Input: part model. Units: mm. Frame: model coordinates. A direction names the side the tool comes from. Round coordinates to 2 decimals unless told otherwise and drop trailing zeros. Put each result on its own line as item: value. Start each with the question number.
1) Reachability of faces 1 (the face through (80, 38.2, -14)), 2 (the face through (137.5, 1, -14)) from +Z, -Z, +X, -X, +Y, -Y: full face, straight path, thin tool, end or side. Return the list, or none.
2) Draft query along Y for faces 3 (the face through (2, 1, -19.5)), 4 (the face through (-80, 41.8, -14)), 5 (the face through (-134.49, 57.15, -13.58)), 6 (the face through (134.49, -57.15, -13.58)). Return one class per face: +Y half, -Y half, draft (parallel to the pull), parting line (faces both ways), or undercut.
3) Line query: probe 1 along Y at (x, z) = (20, -9.75); probe 2 along Y at (x, z) = (80, -16.5); probe 3 along X at (y, z) = (-41, -11.75). Output: solid intervals per line, ascending.
from build123d import *

# Parameters (mm, degrees)
SKETCH001_R  = 1.8
PAD001_DEPTH = 12


with BuildPart() as part:
    # Sketch001 → Pad001 (new body)
    with BuildSketch(Plane.XY.offset(-19.5)):
        with BuildLine():
            Line((-127.5, 60), (127.5, 60))
            ThreePointArc((137.5, 49.999999), (134.571068, 57.071067), (127.5, 60))
            Line((137.5, 49.999999), (137.5, -49.999999))
            ThreePointArc((127.5, -60), (134.571068, -57.071067), (137.5, -49.999999))
            Line((127.5, -60), (-127.5, -60))
            ThreePointArc((-137.5, -50), (-134.571068, -57.071067), (-127.5, -60))
            Line((-137.5, -50), (-137.5, 50))
            ThreePointArc((-127.5, 60), (-134.571068, 57.071068), (-137.5, 50))
        make_face()
        with Locations((-80, -40)):
            Circle(SKETCH001_R, mode=Mode.SUBTRACT)
        with Locations((-50, -40)):
            Circle(SKETCH001_R, mode=Mode.SUBTRACT)
        with Locations((50, -40)):
            Circle(SKETCH001_R, mode=Mode.SUBTRACT)
        with Locations((80, -40)):
            Circle(SKETCH001_R, mode=Mode.SUBTRACT)
        with Locations((-127.5, -50)):
            Circle(SKETCH001_R, mode=Mode.SUBTRACT)
        with Locations((-127.5, 50)):
            Circle(SKETCH001_R, mode=Mode.SUBTRACT)
        with Locations((127.5, 50)):
            Circle(SKETCH001_R, mode=Mode.SUBTRACT)
        with Locations((127.5, -50)):
            Circle(SKETCH001_R, mode=Mode.SUBTRACT)
        with Locations((-20, 20)):
            Circle(SKETCH001_R, mode=Mode.SUBTRACT)
        with Locations((20, 20)):
            Circle(SKETCH001_R, mode=Mode.SUBTRACT)
        with Locations((-20, -20)):
            Circle(SKETCH001_R, mode=Mode.SUBTRACT)
        with Locations((20, -20)):
            Circle(SKETCH001_R, mode=Mode.SUBTRACT)
        with BuildLine():
            ThreePointArc((-82.5, 41.8), (-84.3, 40), (-82.5, 38.2))
            Line((-82.5, 38.2), (-77.5, 38.2))
            ThreePointArc((-77.5, 38.2), (-75.7, 40), (-77.5, 41.8))
            Line((-82.5, 41.8), (-77.5, 41.8))
        make_face(mode=Mode.SUBTRACT)
        with BuildLine():
            ThreePointArc((-52.5, 41.8), (-54.3, 40), (-52.5, 38.2))
            Line((-52.5, 38.2), (-47.5, 38.2))
            ThreePointArc((-47.5, 38.2), (-45.7, 40), (-47.5, 41.8))
            Line((-52.5, 41.8), (-47.5, 41.8))
        make_face(mode=Mode.SUBTRACT)
        with BuildLine():
            ThreePointArc((47.5, 41.8), (45.7, 40), (47.5, 38.2))
            Line((47.5, 38.2), (52.5, 38.2))
            ThreePointArc((52.5, 38.2), (54.3, 40), (52.5, 41.8))
            Line((47.5, 41.8), (52.5, 41.8))
        make_face(mode=Mode.SUBTRACT)
        with BuildLine():
            ThreePointArc((77.5, 41.8), (75.7, 40), (77.5, 38.2))
            Line((77.5, 38.2), (82.5, 38.2))
            ThreePointArc((82.5, 38.2), (84.3, 40), (82.5, 41.8))
            Line((77.5, 41.8), (82.5, 41.8))
        make_face(mode=Mode.SUBTRACT)
    extrude(amount=PAD001_DEPTH)


solid = part.part
Geometry results:
1. face 1: +Z, -Z
1. face 2: +Z, -Z, +X, +Y, -Y
2. face 3: draft
2. face 4: undercut
2. face 5: +Y half
2. face 6: -Y half
3. probe 1: y = -60 to -21.8, -18.2 to 18.2, 21.8 to 60
3. probe 2: y = -60 to -41.8, -38.2 to 38.2, 41.8 to 60
3. probe 3: x = -137.5 to -81.5, -78.5 to -51.5, -48.5 to 48.5, 51.5 to 78.5, 81.5 to 137.5
